from build123d import *

# Parameters (mm, degrees)
EXTRUDE1_DEPTH = 3.048
SKETCH3_R      = 0.3175
EXTRUDE2_DEPTH = 3.81


with BuildPart() as part:
    # Sketch1 → Extrude1 (new, symmetric)
    with BuildSketch(Plane.XY):
        Polygon((0, 0), (0, 6.096), (-4.953, 6.096), (-9.017, 2.032), (-9.017, 0), align=None)
    extrude(amount=EXTRUDE1_DEPTH, both=True)

    # Sketch2 → Revolve1 (revolve)
    with BuildSketch(Plane.XY, mode=Mode.PRIVATE) as revolve1_sk:
        with BuildLine():
            Line((-1.016, 3.048), (5.0038, 3.048))
            ThreePointArc((5.0038, 3.048), (4.297048663, 4.754248663), (2.5908, 5.461))
            Line((2.5908, 5.461), (-1.016, 5.461))
            Line((-1.016, 5.461), (-1.016, 3.048))
        make_face()
    revolve(revolve1_sk.sketch.rotate(Axis((5.0038, 3.048, 0), (1, 0, 0)), 90), axis=Axis((5.0038, 3.048, 0), (1, 0, 0)))

    # Sketch3 → Extrude2 (add)
    with BuildSketch(Plane(origin=(0, 0, 0), x_dir=(1, 0, 0), z_dir=(0, 1, 0))):
        with Locations(Location((-5.207, -1.27, 0), (0, 0, 270))):
            Circle(SKETCH3_R)
        with Locations(Location((-5.207, 1.27, 0), (0, 0, 270))):
            Circle(SKETCH3_R)
    extrude(amount=-EXTRUDE2_DEPTH)


solid = part.part
Design review of the part built by this model. Coordinates are the model's own, in mm. A direction names the side the tool comes from. Coordinates: 2 decimals unless noted, no trailing zeros. Loops run counter-clockwise (first coordinate to the right, second up) from the corner with the lowest first, then second, coordinate; pieces in that order, holes last. Notation, with made-up numbers: (81, 24) -> (114, 24) arc R19 cw to (114, 54) -> close; hole circle Ø9 at (6.25, 27.5). An arc over 180 degrees is marked (long way). Use a Markdown table: item, result. Add a question column.
Item 1: We need section A-A, the plane z = 0. Write out the cut boundary in (x, y) (3 decimals).
Item 2: Clearance check with flat-ended pins moving along their axes: P1, Ø1.8, axis at x = -6.5, z = -0.5, coming from the -Y side; P2, Ø1, axis at y = 0.5, z = -2, coming from the +X side; P3, Ø1.5, axis at y = 3.5, z = 2, coming from the +X side. State where each tip first meets the part, or that it passes through.
Item 3: Machinability: for faces 1 (the flat face through (-6.96, 4.09, 0.04)), 2 (the cylindrical face through (1.28, 4.52, -1.91)), which of the approach directions +Z, -Z, +X, -X, +Y, -Y give a long, thin tool a straight path to every point of the face, cutting with its end or side? Answer none if there is none.
Item 4: Wall thickness on L1, parallel to X at y = 0.5, z = 1.5; L2, parallel to Y at x = -0.75, z = 2.25; L3, parallel to X at y = 5, z = 2.5: over which ranges is each line inside the solid? List them lowest first. Write a range as from..to.
Item 5: We need section D-D, the plane x = -0.25. Write out the cut boundary in (y, z), and give its area (3 significant figures).
Item 6: We need section C-C, the plane y = 1.25. Write out the cut boundary in (x, z).
Item 7: We need section B-B, the plane y = -1.5. Write out the cut boundary in (x, z) (1 decimal).
Numbers:
| question | item | result |
|---|---|---|
| 1 | outline | (-9.017, 0) -> (0, 0) -> (0, 0.635) -> (2.591, 0.635) arc R2.413 ccw to (2.591, 5.461) -> (0, 5.461) -> (0, 6.096) -> (-4.953, 6.096) -> (-9.017, 2.032) -> close |
| 2 | P1 | stops at y = 0 |
| 2 | P2 | stops at x = 0 |
| 2 | P3 | stops at x = 4.62 |
| 3 | face 1 | +Z, -Z, -X, +Y |
| 3 | face 2 | +X |
| 4 | L1 | x = -9.02..0 |
| 4 | L2 | y = 0..6.1 |
| 4 | L3 | x = -6.05..0 |
| 5 | outline | (0, -3.05) -> (6.1, -3.05) -> (6.1, 3.05) -> (0, 3.05) -> close |
| 5 | area | 37.2 mm^2 |
| 6 | outline | (-9.02, -3.05) -> (0, -3.05) -> (0, -1.61) -> (2.59, -1.61) arc R1.61 ccw to (2.59, 1.61) -> (0, 1.61) -> (0, 3.05) -> (-9.02, 3.05) -> close |
| 7 | outline | circle Ø0.6 at (-5.2, -1.3); circle Ø0.6 at (-5.2, 1.3) |
